Geometry: final body of the model. Coordinates: model frame, mm. A direction names the side the tool comes from. Give positions to 0.01 mm unless a question says otherwise; leave off trailing zeros. Write each loop counter-clockwise with the first axis right and the second up, starting at its lowest first coordinate (ties: lowest second). Pieces come first, ordered by that corner, then holes. Notation, with made-up numbers: M -24,-26.5 L 15,-26.5 A4 ccw 15,-20.5 Z; hole C 87.5,78.25 d6. An arc over 180 degrees is marked long. Use a Markdown table: item, result. Add a question column.
(1) Cut plane A-A (y = 12). Output: boundary loops of the cut face in (x, z), plus the area to 3 significant figures.
(2) Cut plane C-C (x = 0). Output: boundary loops of the cut face in (y, z).
(3) Draft query along X for faces 4 (the cylindrical face through (0, 35, -39)), 5 (the cylindrical face through (59, 8, -2)), 6 (the flat face through (20, 8, -39)), 7 (the flat face through (40, 0, -39)). Return one class per face: released by +X, released by -X, zero draft, split by the parting line, or undercut.
(4) Reachability of faces 1 (the flat face through (-47, 15, -39)), 2 (the flat face through (48, 15, -39)), 3 (the flat face through (-20, 7, -39)) from +Z, -Z, +X, -X, +Y, -Y: full face, straight path, thin tool, end or side. Return the list, or none.
(5) Pin query (flat end, axial travel): pin 1 Ø7.5 at (x, z) = (-52.5, -46) entering from +Y; pin 2 Ø1.5 at (x, z) = (12, -16.5) entering from +Y; pin 3 Ø1.5 at (x, z) = (16, -32.5) entering from -Y. Return the tip coordinate at first contact, or that it passes through.
(6) Cut plane B-B (z = -64). Output: boundary loops of the cut face in (x, y), plus the area to 3 significant figures.
(7) Material intervals for L1, parallel to X at y = 6.5, z = -11.5; L2, parallel to X at y = 15.5, z = -4.5; L3, parallel to Y at x = -39.5, z = -37.5, sorted ascending.
(8) Cut plane D-D (y = 31). Output: boundary loops of the cut face in (x, z).
```python
from build123d import *

# Parameters (mm, degrees)
EXTRUDE_1_DEPTH = 80
FILLET_1_R      = 5


with BuildPart() as part:
    # Эскиз1 → Бобышка-Вытянуть1 (new body)
    with BuildSketch(Plane.XY):
        with BuildLine():
            Line((-60, 0), (-20, 0))
            Line((-20, 0), (-20, 15))
            ThreePointArc((-20, 15), (0, 35), (20, 15))
            Line((20, 15), (20, 0))
            Line((20, 0), (60, 0))
            Line((60, 0), (60, 15))
            Line((60, 15), (35, 15))
            ThreePointArc((35, 15), (0, 50), (-35, 15))
            Line((-35, 15), (-60, 15))
            Line((-60, 15), (-60, 0))
        make_face()
    extrude(amount=-EXTRUDE_1_DEPTH)

    # Скругление1
    fillet_1_edges = [part.edges().sort_by_distance(p)[0] for p in [
        (60, 7.5, 0),
        (-60, 7.5, 0),
        (60, 7.5, -80),
        (-60, 7.5, -80),
    ]]
    fillet(fillet_1_edges, radius=FILLET_1_R)


solid = part.part
```
Answer list:
| question | item | result |
|---|---|---|
| 1 | outline | M -60,-75 A5 ccw -55,-80 L -20,-80 L -20,0 L -55,0 A5 ccw -60,-5 Z; M 20,-80 L 55,-80 A5 ccw 60,-75 L 60,-5 A5 ccw 55,0 L 20,0 Z |
| 1 | area | 6,380 mm² |
| 2 | outline | M 35,-80 L 50,-80 L 50,0 L 35,0 Z |
| 3 | face 4 | undercut |
| 3 | face 5 | released by +X |
| 3 | face 6 | undercut |
| 3 | face 7 | zero draft |
| 4 | face 1 | +Z, -Z, -X, +Y |
| 4 | face 2 | +Z, -Z, +X, +Y |
| 4 | face 3 | +Z, -Z, -Y |
| 5 | pin 1 | y = 15 |
| 5 | pin 2 | y = 48.14 |
| 5 | pin 3 | y = 25.93 |
| 6 | outline | M -60,0 L -20,0 L -20,15 A20 cw 20,15 L 20,0 L 60,0 L 60,15 L 35,15 A35 ccw -35,15 L -60,15 Z |
| 6 | area | 2,500 mm² |
| 7 | L1 | -60 to -20, 20 to 60 |
| 7 | L2 | -35 to -19.99, 19.99 to 35 |
| 7 | L3 | 0 to 15 |
| 8 | outline | M -31.13,-80 L -12,-80 L -12,0 L -31.13,0 Z; M 12,-80 L 31.13,-80 L 31.13,0 L 12,0 Z |
